Model file for the job. Use its own axes, mm. A direction names the side the tool comes from. Coordinates: 2 decimals unless noted, no trailing zeros. Loops run counter-clockwise (first coordinate to the right, second up) from the corner with the lowest first, then second, coordinate; pieces in that order, holes last. Notation, with made-up numbers: M -28.5,-27 L -21.5,-27 A27 cw -21.5,-4 Z; hole C 37,60 d8. An arc over 180 degrees is marked long. Write item = value, one per line. Start each with the question number.
from build123d import *

# Parameters (mm, degrees)
EXTRUDE_1_DEPTH = 9
SKETCH_2_R      = 1.6
EXTRUDE_2_DEPTH = 4
FILLET_1_R      = 4
FILLET_2_R      = 1.6
CHAMFER_1_SIZE  = 0.2


with BuildPart() as part:
    # 草图1 → 凸台-拉伸1 (new body)
    with BuildSketch(Plane(origin=(0, 0, 0), x_dir=(1, 0, 0), z_dir=(0, 1, 0))):
        Polygon((106.5, 0), (0, 0), (0, -4), (114.5, -4), (114.5, 28), (0, 28), (0, 24), (106.5, 24), (106.5, 16.6), (110.5, 16.6), (110.5, 7.4), (106.5, 7.4), align=None)
    extrude(amount=EXTRUDE_1_DEPTH)

    # 草图2 → 凸台-拉伸2 (add)
    # profile 1 of 2: a face of its own
    with BuildSketch(Plane.ZY):
        with BuildLine():
            Line((8.5, 9), (4, 9))
            Line((4, 9), (4, 0))
            Line((4, 0), (8.5, 0))
            ThreePointArc((8.5, 0), (13, 4.5), (8.5, 9))
        make_face()
        with Locations((8.5, 4.5)):
            Circle(SKETCH_2_R, mode=Mode.SUBTRACT)
    # profile 2 of 2: a face of its own
    with BuildSketch(Plane.ZY):
        with BuildLine():
            Line((-28, 0), (-28, 9))
            Line((-28, 9), (-32.5, 9))
            ThreePointArc((-32.5, 9), (-37, 4.5), (-32.5, 0))
            Line((-32.5, 0), (-28, 0))
        make_face()
        with Locations((-32.5, 4.5)):
            Circle(SKETCH_2_R, mode=Mode.SUBTRACT)
    extrude(amount=-EXTRUDE_2_DEPTH)

    # 圆角1
    fillet_1_edges = [part.edges().sort_by_distance(p)[0] for p in [
        (0, 4.5, -24),
        (114.5, 4.5, -28),
        (114.5, 4.5, 4),
        (0, 4.5, 0),
    ]]
    fillet(fillet_1_edges, radius=FILLET_1_R)

    # 圆角2
    fillet_2_edges = [part.edges().sort_by_distance(p)[0] for p in [
        (106.5, 4.5, -16.6),
        (106.5, 4.5, -24),
        (106.5, 4.5, 0),
        (106.5, 4.5, -7.4),
        (4, 4.5, -28),
        (4, 4.5, 4),
    ]]
    fillet(fillet_2_edges, radius=FILLET_2_R)

    # 倒角1
    chamfer_1_edges = [part.edges().sort_by_distance(p)[0] for p in [
        (106.5, 0, -3.7),
        (106.5, 9, -3.7),
        (58.05, 0, -28),
        (58.05, 0, 4),
        (54.45, 0, 0),
        (106.5, 0, -20.3),
        (106.96862915, 0, -17.06862915),
        (106.96862915, 0, -6.93137085),
        (58.05, 9, -28),
        (4, 9, -31.05),
        (106.5, 9, -20.3),
        (54.45, 9, 0),
        (4, 9, 7.05),
        (58.05, 9, 4),
        (106.96862915, 9, -17.06862915),
        (106.96862915, 9, -6.93137085),
        (109.3, 9, -7.4),
        (106.03137085, 0, -0.46862915),
        (106.03137085, 9, -0.46862915),
        (4.46862915, 9, 4.46862915),
        (4.46862915, 0, 4.46862915),
        (4.46862915, 0, -28.46862915),
        (4.46862915, 9, -28.46862915),
        (106.03137085, 0, -23.53137085),
        (106.03137085, 9, -23.53137085),
        (109.3, 0, -7.4),
        (110.5, 0, -12),
        (109.3, 0, -16.6),
        (109.3, 9, -16.6),
        (0, 4.5, -37),
        (4, 0, -31.05),
        (4, 4.5, -37),
        (4, 4.5, 13),
        (4, 0, 7.05),
        (0, 4.5, 13),
        (54.45, 0, -24),
        (0, 0, -30.25),
        (114.5, 0, -12),
        (0, 0, 6.25),
        (1.171572875, 0, -25.171572875),
        (1.171572875, 0, 1.171572875),
        (113.328427125, 0, 2.828427125),
        (113.328427125, 0, -26.828427125),
        (114.5, 9, -12),
        (110.5, 9, -12),
        (0, 9, 6.25),
        (0, 9, -30.25),
        (54.45, 9, -24),
        (1.171572875, 9, -25.171572875),
        (1.171572875, 9, 1.171572875),
        (113.328427125, 9, 2.828427125),
        (113.328427125, 9, -26.828427125),
    ]]
    chamfer(chamfer_1_edges, length=CHAMFER_1_SIZE)


solid = part.part
Item 1: 3-axis set-ups, long thin cutter, end or side, ignore diameter. For faces 1 (the cylindrical face through (2, 4.4, 13)), 2 (the flat face through (109, 4, -7.4)), 3 (the flat face through (57, 4, 4)): which of +Z, -Z, +X, -X, +Y, -Y reach the whole face in a straight line?
Item 2: Pull direction Z, two halves, no side cores. Call faces 4 (the cylindrical face through (2, 4.6, -37)), 5 (the flat face through (54, 4, -24)), 6 (the cylindrical face through (113.359, 4.56, 2.797)), 7 (the flat face through (4, 3.6, -34.1)): +Z half, -Z half, draft (parallel to the pull), parting line (faces both ways), or undercut.
Item 3: Cut at B-B (z = -15). Give the cut face in (x, y), plus the area to 3 significant figures.
Item 4: Cut at C-C (y = 4.5). Give the number of separate pieces and of enclosed holes in the cut face, plus the area to 3 significant figures.
Item 5: Cut at A-A (x = 52). Give the cut face in (y, z).
Item 6: Pin check, flat tips, straight feed: pin 1 Ø3.5 at (y, z) = (5, 9) entering from +X; pin 2 Ø1 at (y, z) = (6, 4) entering from +X; pin 3 Ø1.9 at (x, y) = (108.5, 3) entering from -Z. Stop position of each tip, or through.
Item 7: Probe L1, parallel to Z at x = 51, y = 2.5; L2, parallel to Y at x = 2.4, z = -32.5; L3, parallel to X at y = 0.5, z = 10. List the from-to ranges inside material, lowest first.
Reported:
q1.face_1 = +Z, +X, -X
q1.face_2 = -X, +Y, -Y
q1.face_3 = +Z, +X, +Y, -Y
q2.face_4 = -Z half
q2.face_5 = undercut
q2.face_6 = +Z half
q2.face_7 = draft
q3.outline = M 110.5,0.2 L 110.7,0 L 114.3,0 L 114.5,0.2 L 114.5,8.8 L 114.3,9 L 110.7,9 L 110.5,8.8 Z
q3.area = 35.9 mm^2
q4.separate_pieces = 3
q4.enclosed_holes = 0
q4.area = 1,100 mm^2
q5.outline = M 0,-27.8 L 0.2,-28 L 8.8,-28 L 9,-27.8 L 9,-24.2 L 8.8,-24 L 0.2,-24 L 0,-24.2 Z; M 0,0.2 L 0.2,0 L 8.8,0 L 9,0.2 L 9,3.8 L 8.8,4 L 0.2,4 L 0,3.8 Z
q6.pin_1 = 4
q6.pin_2 = 112.44
q6.pin_3 = -28
q7.L1 = -28 to -24, 0 to 4
q7.L2 = 0 to 2.9, 6.1 to 9
q7.L3 = 0 to 4
